```python
from build123d import *

# Parameters (mm, degrees)
BOSS_EXTRUDE2_DEPTH = 5


with BuildPart() as part:
    # Sketch1 → Boss-Extrude2 (new body, symmetric)
    with BuildSketch(Plane.XY):
        with BuildLine():
            Line((-11.5, -108.94), (-125, -108.94))
            Line((-125, -108.94), (-125, 108.94))
            Line((-125, 108.94), (-54.45, 193.35))
            Line((-54.45, 193.35), (54.45, 193.35))
            Line((54.45, 193.35), (125, 108.94))
            Line((125, 108.94), (125, -108.94))
            Line((125, -108.94), (11.5, -108.94))
            ThreePointArc((11.5, -108.94), (0, -97.44), (-11.5, -108.94))
        make_face()
    extrude(amount=BOSS_EXTRUDE2_DEPTH, both=True)


solid = part.part
```
For this review, take the finished solid that the model builds, in its own axes (mm). Coordinates: 2 decimals unless noted, no trailing zeros. Loops run counter-clockwise (first coordinate to the right, second up) from the corner with the lowest first, then second, coordinate; pieces in that order, holes last.
1. For line 1 (X direction, y = 152.5, z = -0.25); line 2 (X direction, y = 121, z = 2); line 3 (Y direction, x = 105.5, z = -2.5), list the stretches that pass through material, from the lowest coordinate up.
2. Insertion check: P1, Ø5, axis at y = 148.5, z = -0.5, coming from the -X side. The pin has a flat end and moves straight along its axis. Give the tip position at first contact, or say it passes through.
3. Add section A-A, the plane z = -1.25. Give the boundary of the cut face in (x, y), then the cut area to 3 significant figures.
4. Add section C-C, the plane x = 75.5. Give the boundary of the cut face in (y, z).
5. Add section B-B, the plane x = 0. Give the boundary of the cut face in (y, z), then the cut area to 3 significant figures.
Result:
1. line 1: x = -88.59 to 88.59
1. line 2: x = -114.92 to 114.92
1. line 3: y = -108.94 to 132.27
2. P1: stops at x = -94.03
3. outline: (-125, -108.94) - (-11.5, -108.94) arc R11.5 cw to (11.5, -108.94) - (125, -108.94) - (125, 108.94) - (54.45, 193.35) - (-54.45, 193.35) - (-125, 108.94) - close
3. area: 69,400 mm2
4. outline: (-108.94, -5) - (168.16, -5) - (168.16, 5) - (-108.94, 5) - close
5. outline: (-97.44, -5) - (193.35, -5) - (193.35, 5) - (-97.44, 5) - close
5. area: 2,910 mm2
